```python
from build123d import *

# Parameters (mm, degrees)
SKETCH_1_R          = 5.5
SKETCH_1_R_2        = 2.5
EXTRUDE_1_DEPTH     = 2.5
SKETCH_3_R          = 6.25
SKETCH_3_R_2        = 2.5
EXTRUDE_2_DEPTH     = 1
SKETCH_4_R          = 5.1
SKETCH_4_R_2        = 2.9
CUT_EXTRUDE_1_DEPTH = 0.2
CHAMFER_1_SIZE      = 0.05


with BuildPart() as part:
    # 草图1 → 凸台-拉伸1 (new body, symmetric)
    with BuildSketch(Plane.XY):
        Circle(SKETCH_1_R)
        Circle(SKETCH_1_R_2, mode=Mode.SUBTRACT)
    extrude(amount=EXTRUDE_1_DEPTH, both=True)

    # 草图3 → 凸台-拉伸2 (add)
    with BuildSketch(Plane(origin=(0, 0, -2.5), x_dir=(-1, 0, 0), z_dir=(0, 0, -1))):
        Circle(SKETCH_3_R)
        Circle(SKETCH_3_R_2, mode=Mode.SUBTRACT)
    extrude(amount=-EXTRUDE_2_DEPTH)

    # 草图4 → 切除-拉伸1 (cut)
    with BuildSketch(Plane.XY.offset(2.5)):
        Circle(SKETCH_4_R)
        Circle(SKETCH_4_R_2, mode=Mode.SUBTRACT)
    cut_extrude_1 = extrude(amount=-CUT_EXTRUDE_1_DEPTH, mode=Mode.SUBTRACT)

    # 镜向1: 切除-拉伸1 across plane
    add(cut_extrude_1.mirror(Plane.XY), mode=Mode.SUBTRACT)

    # 倒角1
    chamfer_1_edges = [part.edges().sort_by_distance(p)[0] for p in [
        (-5.1, 0, 2.5),
        (-2.9, 0, 2.5),
        (-2.9, 0, -2.5),
        (-5.1, 0, -2.5),
        (-5.5, 0, 2.5),
        (-2.5, 0, -2.5),
        (-2.5, 0, 2.5),
    ]]
    chamfer(chamfer_1_edges, length=CHAMFER_1_SIZE)


solid = part.part
```
Check sheet for the modelled part. Datum: model origin and axes. Units: mm. A direction names the side the tool comes from. Round coordinates to 2 decimals unless told otherwise and drop trailing zeros. Loops run counter-clockwise (first coordinate to the right, second up) from the corner with the lowest first, then second, coordinate; pieces in that order, holes last. Notation, with made-up numbers: (-8, -22) - (-2, -22) arc R18 ccw to (-2, -15) - close; hole circle Ø7 at (-40, -11). An arc over 180 degrees is marked (long way). Write item = value, one per line. Start each with the question number.
Q1. Access from +Z, -Z, +X, -X, +Y, -Y to the whole of each face (thin tool, end or side, straight path). Record for faces 1 (the face through (-0.54, -2.44, -0.03)), 2 (the face through (0, -6, -1.5)).
Q2. Thickness scan on L1, parallel to Y at x = 0, z = 2.4; L2, parallel to X at y = 0.5, z = 2.35; L3, parallel to Z at x = 4.25, y = -0.25. Record the ranges inside material, lowest first.
Q3. Section check A-A (z = 1.75). Record the boundary of the cut face in (x, y).
Q4. Depth check by flat-ended pin: P1, Ø6, axis at x = 3.5, y = -2, coming from the -Z side; P2, Ø2, axis at y = 4, z = 0, coming from the +X side. Enter the tip coordinate at first touch or a pass-through.
Q5. Release check for a two-part mould opening along X. For faces 3 (the face through (-5.96, 1.88, -2.01)), 4 (the face through (2.2, -2.2, -2.3)), 5 (the face through (2.2, -2.2, 2.3)), 6 (the face through (2, 5, -2.5)) record: pulls with the +X half, pulls with the -X half, needs draft (parallel to the pull), parting line crosses it, or undercut.
Derived:
q1.face_1 = +Z, -Z
q1.face_2 = +Z
q2.L1 = -5.5 to -5.1, -2.9 to -2.5, 2.5 to 2.9, 5.1 to 5.5
q2.L2 = -5.48 to -5.08, -2.86 to -2.45, 2.45 to 2.86, 5.08 to 5.48
q2.L3 = -2.3 to 2.3
q3.outline = circle Ø11 at (0, 0); hole circle Ø5 at (0, 0)
q4.P1 = -2.5
q4.P2 = 4.61
q5.face_3 = parting line crosses it
q5.face_4 = undercut
q5.face_5 = undercut
q5.face_6 = needs draft
